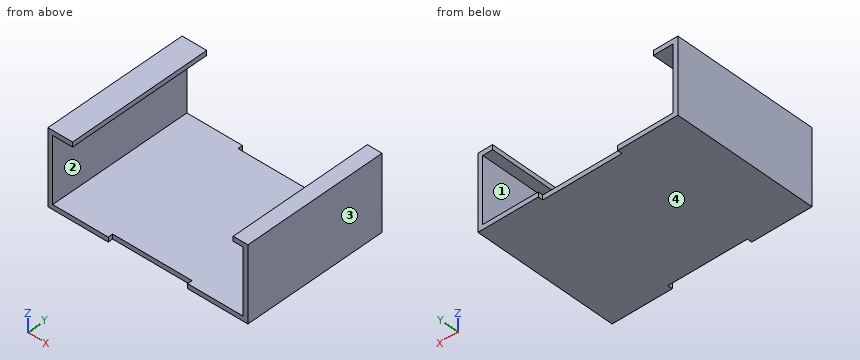
```python
from build123d import *

# Parameters (mm, degrees)
F1_DEPTH = 1.2
F0_W     = 1.2
F0_H     = 36.5
F2_DEPTH = 17.7
F3_W     = 1.2
F3_H     = 36.5
F3_W_2   = 5
F3_W_3   = 3.7
F4_DEPTH = 1.2


with BuildPart() as f1:
    # F0 (on Top) → F1 (new body)
    with BuildSketch(Plane.XY):
        Polygon((10, -18.25), (24, -18.25), (24, 18.25), (10, 18.25), (10, 17.05), (-10, 17.05), (-10, 18.25), (-24, 18.25), (-24, -18.25), (-10, -18.25), (-10, -17.05), (10, -17.05), align=None)
    extrude(amount=F1_DEPTH)

    # F0 (on Top) → F2 (join)
    with BuildSketch(Plane.XY):
        with Locations((-24.6, 0)):
            Rectangle(F0_W, F0_H)
        with Locations((24.6, 0)):
            Rectangle(F0_W, F0_H)
    extrude(amount=F2_DEPTH)

    # F3 (on face) → F4 (join)
    with BuildSketch(Plane.XY.offset(17.7)):
        with Locations((-24.6, 0)):
            Rectangle(F3_W, F3_H)
        with Locations((-21.5, 0)):
            Rectangle(F3_W_2, F3_H)
        with Locations((23.35, 0)):
            Rectangle(F3_W_3, F3_H)
    extrude(amount=F4_DEPTH)


solid = f1.part
```
Input: part model. Units: mm. Frame: model coordinates. Face numbers are marked on the shaded views. Round coordinates to 2 decimals unless told otherwise and drop trailing zeros. Loops run counter-clockwise (first coordinate to the right, second up) from the corner with the lowest first, then second, coordinate; pieces in that order, holes last. Notation, with made-up numbers: M 22.5,-24.5 L 36.5,-24.5 A8 cw 36.5,-14.5 Z; hole C 79.25,56.5 d7. An arc over 180 degrees is marked long. Answer in a Markdown table with one row per item. Add a question column.
1. Section C-C (x = -0.5). Output: boundary loops of the cut face in (y, z).
2. Section D-D (x = -12). Output: boundary loops of the cut face in (y, z).
3. Mould query, pull axis Z, two halves, no side actions, for the marked faces 1, 2, 3 and 4. Classes: released by +Z, released by -Z, zero draft, split by the parting line, or undercut.
4. Section A-A (z = 11.25). Output: boundary loops of the cut face in (x, y).
5. Contact query for flat-ended pins moving along their axis: pin 1 (1 mm diameter, centred on x = -1.5, z = 0.5, fed in from -Y); pin 2 (2 mm diameter, centred on x = 1.5, y = 0, fed in from +Z). Output: stop coordinate, or through.
6. Ray query, probe 1 along X at (y, z) = (0.5, 3.25); probe 2 along Z at (x, y) = (22.5, 5.5); probe 3 along Z at (x, y) = (-17, 15.5). Return the intervals inside material, ascending.
7. Section B-B (y = -5.5). Output: boundary loops of the cut face in (x, z).
Values follow:
| question | item | result |
|---|---|---|
| 1 | outline | M -17.05,0 L 17.05,0 L 17.05,1.2 L -17.05,1.2 Z |
| 2 | outline | M -18.25,0 L 18.25,0 L 18.25,1.2 L -18.25,1.2 Z |
| 3 | face 1 | undercut |
| 3 | face 2 | undercut |
| 3 | face 3 | zero draft |
| 3 | face 4 | released by -Z |
| 4 | outline | M -25.2,-18.25 L -24,-18.25 L -24,18.25 L -25.2,18.25 Z; M 24,-18.25 L 25.2,-18.25 L 25.2,18.25 L 24,18.25 Z |
| 5 | pin 1 | y = -17.05 |
| 5 | pin 2 | z = 1.2 |
| 6 | probe 1 | -25.2 to -24, 24 to 25.2 |
| 6 | probe 2 | 0 to 1.2, 17.7 to 18.9 |
| 6 | probe 3 | 0 to 1.2 |
| 7 | outline | M -25.2,0 L 25.2,0 L 25.2,18.9 L 21.5,18.9 L 21.5,17.7 L 24,17.7 L 24,1.2 L -24,1.2 L -24,17.7 L -19,17.7 L -19,18.9 L -25.2,18.9 Z |
